Can you work these out from the model? Positions are in its coordinate system, mm. A direction names the side the tool comes from. Coordinates: 2 decimals unless noted, no trailing zeros. Order: outer loops, then holes, each group sorted by start corner. A loop starts at its lowest first (then second) coordinate and runs counter-clockwise, first axis right, second up. Notation, with made-up numbers: (31, 0.5) -> (37, 0.5) arc R16 ccw to (37, 18.5) -> close; hole circle Ø9 at (-8.5, 3). An arc over 180 degrees is marked (long way). Answer in a Markdown table with one row per item.
```python
from build123d import *
from build123d.topology import SkipClean

# Parameters (mm, degrees)
SKETCH1_R               = 21
BOSS_EXTRUDE1_DEPTH     = 1.5
SKETCH2_R               = 2.65
CUT_EXTRUDE1_DEPTH      = 1.5
SKETCH5_W               = 10
SKETCH5_H               = 50
BOSS_EXTRUDE2_DEPTH     = 1.5
CIRPATTERN1_DEPTH       = 1.5
CUT_EXTRUDE4_REACH      = 56.252
SKETCH4_R               = 1.65
CUT_EXTRUDE5_REACH      = 56.314
SKETCH6_R               = 1.5
CUT_EXTRUDE6_DEPTH      = 55.251728083
CUT_EXTRUDE6_DEPTH_BACK = 55.251728083
CUT_EXTRUDE8_REACH      = 56.18
SKETCH9_R               = 1.5


# Read off the part's stored shape, not the designer's step: CirPattern1
with BuildPart() as part:
    # Sketch1 → Boss-Extrude1 (new, symmetric)
    with BuildSketch(Plane(origin=(0, 0, 0), x_dir=(1, 0, 0), z_dir=(0, 1, 0))):
        with Locations(Location((0, 0, 0), (0, 0, 270))):
            Circle(SKETCH1_R)
    extrude(amount=BOSS_EXTRUDE1_DEPTH, both=True)

    # Sketch2 → Cut-Extrude1 (cut)
    with BuildSketch(Plane(origin=(0, 1.5, 0), x_dir=(1, 0, 0), z_dir=(0, 1, 0))):
        with Locations((0, -15)):
            Circle(SKETCH2_R)
        with BuildLine():
            ThreePointArc((-2.65, -15), (0, -12.35), (2.65, -15))
            Line((2.65, -15), (4.067821782, -0.821782178))
            ThreePointArc((4.067821782, -0.821782178), (0, -4.15), (-4.067821782, -0.821782178))
            Line((-4.067821782, -0.821782178), (-2.65, -15))
        make_face()
        with BuildLine():
            ThreePointArc((-4.067821782, -0.821782178), (0, -4.15), (4.067821782, -0.821782178))
            Line((4.067821782, -0.821782178), (4.15, 0))
            ThreePointArc((4.15, 0), (0, 4.15), (-4.15, 0))
            Line((-4.15, 0), (-4.067821782, -0.821782178))
        make_face()
    cut_extrude1 = extrude(amount=-CUT_EXTRUDE1_DEPTH, mode=Mode.SUBTRACT)

    # Sketch5 → Boss-Extrude2 (add, symmetric)
    with BuildSketch(Plane(origin=(0, 0, 0), x_dir=(1, 0, 0), z_dir=(0, 1, 0))):
        with Locations((0, -25)):
            Rectangle(SKETCH5_W, SKETCH5_H)
    extrude(amount=BOSS_EXTRUDE2_DEPTH, both=True)

    # Mirror1: Cut-Extrude1 across plane
    with SkipClean():  # the faces are left unmerged after this step: merging them gives an invalid solid
        add(cut_extrude1.mirror(Plane.XY), mode=Mode.SUBTRACT)

    # CirPattern1 outline → CirPattern1 (cut)
    with BuildSketch(Plane(origin=(0, 0, 0), x_dir=(1, 0, 0), z_dir=(0, 1, 0))):
        with BuildLine():
            Line((3.772727273, -3.772727273), (15, -2.65))
            ThreePointArc((15, -2.65), (17.65, 0), (15, 2.65))
            Line((15, 2.65), (3.772727273, 3.772727273))
            Line((3.772727273, 3.772727273), (4.067821782, 0.821782178))
            ThreePointArc((4.067821782, 0.821782178), (0, -4.15), (-4.067821782, 0.821782178))
            Line((-4.067821782, 0.821782178), (-3.772727273, 3.772727273))
            Line((-3.772727273, 3.772727273), (-15, 2.65))
            ThreePointArc((-15, 2.65), (-17.65, 0), (-15, -2.65))
            Line((-15, -2.65), (-3.772727273, -3.772727273))
            Line((-3.772727273, -3.772727273), (-2.65, -15))
            ThreePointArc((-2.65, -15), (0, -17.65), (2.65, -15))
            Line((2.65, -15), (3.772727273, -3.772727273))
        make_face()
    extrude(amount=CIRPATTERN1_DEPTH, mode=Mode.SUBTRACT)

    # Sketch4 → Cut-Extrude4 (cut, up to next)
    with BuildSketch(Plane(origin=(0, 0, 0), x_dir=(1, 0, 0), z_dir=(0, 1, 0)), mode=Mode.PRIVATE) as cut_extrude4_sk1:
        with Locations(Location((0, 0, 0), (0, 0, 270))):
            Circle(SKETCH4_R)
    cut_extrude4_tool1 = extrude(cut_extrude4_sk1.sketch, amount=-CUT_EXTRUDE4_REACH, mode=Mode.PRIVATE) & part.part
    add(cut_extrude4_tool1.solids().sort_by_distance((0, 0, 0))[0], mode=Mode.SUBTRACT)

    # Sketch6 → Cut-Extrude5 (cut, up to next)
    with BuildSketch(Plane(origin=(0, 1.5, 0), x_dir=(1, 0, 0), z_dir=(0, 1, 0)), mode=Mode.PRIVATE) as cut_extrude5_sk1:
        with Locations(Location((2.5, -45.5, 0), (0, 0, 270))):
            Circle(SKETCH6_R)
    cut_extrude5_tool1 = extrude(cut_extrude5_sk1.sketch, amount=-CUT_EXTRUDE5_REACH, mode=Mode.PRIVATE) & part.part
    # Sketch6 → Cut-Extrude5 (cut, up to next)
    with BuildSketch(Plane(origin=(0, 1.5, 0), x_dir=(1, 0, 0), z_dir=(0, 1, 0)), mode=Mode.PRIVATE) as cut_extrude5_sk2:
        with Locations(Location((-2.5, -45.5, 0), (0, 0, 270))):
            Circle(SKETCH6_R)
    cut_extrude5_tool2 = extrude(cut_extrude5_sk2.sketch, amount=-CUT_EXTRUDE5_REACH, mode=Mode.PRIVATE) & part.part
    add(cut_extrude5_tool1.solids().sort_by_distance((2.5, 1.5, 45.5))[0], mode=Mode.SUBTRACT)
    add(cut_extrude5_tool2.solids().sort_by_distance((-2.5, 1.5, 45.5))[0], mode=Mode.SUBTRACT)

    # Sketch7 → Cut-Extrude6 (cut, two sides: drawn at the far end of the back side and taken through both)
    with BuildSketch(Plane(origin=(0, 0, 0), x_dir=(1, 0, 0), z_dir=(0, 1, 0)).offset(-CUT_EXTRUDE6_DEPTH_BACK)):
        with BuildLine():
            ThreePointArc((5, -20.396078054), (0, 21), (-5, -20.396078054))
            Line((-5, -20.396078054), (-5.519486194, -16.207382355))
            ThreePointArc((-5.519486194, -16.207382355), (-5.607043009, -15.695391034), (-5.647210443, -15.177522436))
            Line((-5.647210443, -15.177522436), (-6.513602442, -6.513602442))
            Line((-6.513602442, -6.513602442), (-15.177522436, -5.647210443))
            ThreePointArc((-15.177522436, -5.647210443), (-20.65, 0), (-15.177522436, 5.647210443))
            Line((-15.177522436, 5.647210443), (-6.513602442, 6.513602442))
            Line((-6.513602442, 6.513602442), (-5.647210443, 15.177522436))
            ThreePointArc((-5.647210443, 15.177522436), (0, 20.65), (5.647210443, 15.177522436))
            Line((5.647210443, 15.177522436), (6.513602442, 6.513602442))
            Line((6.513602442, 6.513602442), (15.177522436, 5.647210443))
            ThreePointArc((15.177522436, 5.647210443), (20.65, 0), (15.177522436, -5.647210443))
            Line((15.177522436, -5.647210443), (6.513602442, -6.513602442))
            Line((6.513602442, -6.513602442), (5.647210443, -15.177522436))
            ThreePointArc((5.647210443, -15.177522436), (5.607043009, -15.695391034), (5.519486194, -16.207382355))
            Line((5.519486194, -16.207382355), (5, -20.396078054))
        make_face()
    extrude(amount=CUT_EXTRUDE6_DEPTH + CUT_EXTRUDE6_DEPTH_BACK, mode=Mode.SUBTRACT)

    # Sketch9 → Cut-Extrude8 (cut, up to next)
    with BuildSketch(Plane(origin=(0, 1.5, 0), x_dir=(1, 0, 0), z_dir=(0, 1, 0)), mode=Mode.PRIVATE) as cut_extrude8_sk1:
        with Locations(Location((0, -25, 0), (0, 0, 270))):
            Circle(SKETCH9_R)
    cut_extrude8_tool1 = extrude(cut_extrude8_sk1.sketch, amount=-CUT_EXTRUDE8_REACH, mode=Mode.PRIVATE) & part.part
    add(cut_extrude8_tool1.solids().sort_by_distance((0, 1.5, 25))[0], mode=Mode.SUBTRACT)


solid = part.part
```
(1) Suppose I cut it at D-D (z = 0). Please give me the cut outline in (x, y).
Response values:
| item | result |
|---|---|
| outline | (-20.65, -1.5) -> (-1.65, -1.5) -> (-1.65, 0) -> (-17.65, 0) -> (-17.65, 1.5) -> (-20.65, 1.5) -> close; (1.65, -1.5) -> (20.65, -1.5) -> (20.65, 1.5) -> (17.65, 1.5) -> (17.65, 0) -> (1.65, 0) -> close |
(2) I need wall thicknesses on line 1 (X direction, y = -0.1, z = 45.5); line 2 (Y direction, x = -13, z = 1.5); line 3 (X direction, y = -1.1, z = 0). Which ranges of each line are inside material? Lowest first, please. Write a range as [from, to].
Response values:
| item | result |
|---|---|
| line 1 | [-5, -4], [-1, 1], [4, 5] |
| line 2 | [-1.5, 0] |
| line 3 | [-20.65, -1.65], [1.65, 20.65] |
(3) Suppose I cut it at A-A (z = 25). Please give me the cut outline in (x, y), and give its area (3 significant figures).
Response values:
| item | result |
|---|---|
| outline | (-5, -1.5) -> (-1.5, -1.5) -> (-1.5, 1.5) -> (-5, 1.5) -> close; (1.5, -1.5) -> (5, -1.5) -> (5, 1.5) -> (1.5, 1.5) -> close |
| area | 21.0 mm2 |
(4) Suppose I cut it at C-C (x = 10.5). Please give me the cut outline in (y, z).
Response values:
| item | result |
|---|---|
| outline | (-1.5, -6.11) -> (1.5, -6.11) -> (1.5, -3.1) -> (0, -3.1) -> (0, 3.1) -> (1.5, 3.1) -> (1.5, 6.11) -> (-1.5, 6.11) -> close |
(5) On a 3-axis mill with a long thin cutter (end or side, diameter ignored), from which of +Z, -Z, +X, -X, +Y, -Y can I reach the whole of each face in a straight line? I mean faces 1 (the cylindrical face through (-0.06, 0.76, -17.65)), 2 (the flat face through (5, 0, 35)), 3 (the flat face through (3, 1.5, 15)), 4 (the cylindrical face through (2.57, 0.02, 44)), 5 (the flat face through (-5, 0, 35)). Say none if no direction works.
Response values:
| item | result |
|---|---|
| face 1 | +Y |
| face 2 | +Z, +X, +Y, -Y |
| face 3 | +Z, -Z, +X, -X, +Y |
| face 4 | +Y, -Y |
| face 5 | +Z, -X, +Y, -Y |
(6) Will these pins go through, and if not, where does the flat tip stop? pin 1 Ø4.5 at (x, z) = (0, 0) entering from +Y; pin 2 Ø1.5 at (y, z) = (0, 41.5) entering from -X.
Response values:
| item | result |
|---|---|
| pin 1 | y = 0 |
| pin 2 | x = -5 |
(7) We'd pull the mould along Z, two halves only. Please class faces 6 (the flat face through (0, 0, 50)), 7 (the flat face through (10.785, -0.021, -6.086)), 8 (the flat face through (-3.22, 0.76, -9.31)): +Z half, -Z half, draft (parallel to the pull), parting line (faces both ways), or undercut.
Response values:
| item | result |
|---|---|
| face 6 | +Z half |
| face 7 | -Z half |
| face 8 | undercut |
